Read the model definition and answer for the solid it produces. Units are mm, in the model's axes. Face numbers are marked on the shaded views. A direction names the side the tool comes from. Coordinates: 2 decimals unless noted, no trailing zeros. Write each loop counter-clockwise with the first axis right and the second up, starting at its lowest first coordinate (ties: lowest second). Pieces come first, ordered by that corner, then holes. Notation, with made-up numbers: (43, -6) -> (68, -6) arc R10 ccw to (68, 10) -> close; hole circle Ø6 at (18.5, 40). An arc over 180 degrees is marked (long way). Return JSON: item names as keys, results as strings.
from build123d import *

# Parameters (mm, degrees)
SKETCH1_W           = 58
SKETCH1_H           = 40
BOSS_EXTRUDE1_DEPTH = 22.5
SKETCH2_W           = 8.5
SKETCH2_H           = 17
SKETCH2_R           = 2.15
BOSS_EXTRUDE2_DEPTH = 4.35
FILLET1_R           = 8


with BuildPart() as part:
    # Sketch1 → Boss-Extrude1 (new body)
    with BuildSketch(Plane(origin=(0, 0, 0), x_dir=(1, 0, 0), z_dir=(0, 1, 0))):
        with Locations((29, -20)):
            Rectangle(SKETCH1_W, SKETCH1_H)
    extrude(amount=BOSS_EXTRUDE1_DEPTH)

    # Sketch2 → Boss-Extrude2 (add)
    # profile 1 of 2: a face of its own
    with BuildSketch(Plane(origin=(0, 22.5, 0), x_dir=(1, 0, 0), z_dir=(0, 1, 0))):
        with Locations((62.25, -20)):
            Rectangle(SKETCH2_W, SKETCH2_H)
        with Locations(Location((62.1, -20, 0), (0, 0, 270))):
            Circle(SKETCH2_R, mode=Mode.SUBTRACT)
    # profile 2 of 2: a face of its own
    with BuildSketch(Plane(origin=(0, 22.5, 0), x_dir=(1, 0, 0), z_dir=(0, 1, 0))):
        with Locations((-4.25, -20)):
            Rectangle(SKETCH2_W, SKETCH2_H)
        with Locations(Location((-4.2, -20, 0), (0, 0, 270))):
            Circle(SKETCH2_R, mode=Mode.SUBTRACT)
    extrude(amount=-BOSS_EXTRUDE2_DEPTH)

    # Fillet1
    fillet1_edges = [part.edges().sort_by_distance(p)[0] for p in [
        (66.5, 20.325, 11.5),
        (66.5, 20.325, 28.5),
        (-8.5, 20.325, 28.5),
        (-8.5, 20.325, 11.5),
    ]]
    fillet(fillet1_edges, radius=FILLET1_R)


solid = part.part
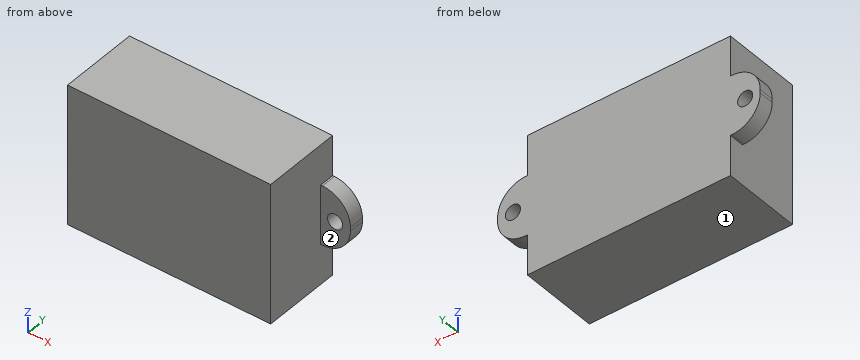
1. The part is cut by section A-A (x = -4.2). Determine the outline of the cut face in (y, z), then the cut area to 3 significant figures.
Taken from the geometry:
{"outline": "(18.15, 12.41) -> (22.5, 12.41) -> (22.5, 17.85) -> (18.15, 17.85) -> close; (18.15, 22.15) -> (22.5, 22.15) -> (22.5, 27.59) -> (18.15, 27.59) -> close", "area": "47.4 mm2"}
2. A tool of negligible diameter and unlimited length cuts with its end or side. For the marked faces 1 and 2, from which of +Z, -Z, +X, -X, +Y, -Y can it reach the whole face along a straight path? Write none if from no direction.
Taken from the geometry:
{"face 1": "-Z, +X, -X, +Y, -Y", "face 2": "+Z, -Z, +X, -Y"}
3. The part is cut by section B-B (z = 13.5). Determine the outline of the cut face in (x, y), then the cut area to 3 significant figures.
Taken from the geometry:
{"outline": "(-5.79, 18.15) -> (0, 18.15) -> (0, 0) -> (58, 0) -> (58, 18.15) -> (63.79, 18.15) -> (63.79, 22.5) -> (-5.79, 22.5) -> close", "area": "1,360 mm2"}
4. The part is cut by section C-C (x = 62.1). Determine the outline of the cut face in (y, z), then the cut area to 3 significant figures.
Taken from the geometry:
{"outline": "(18.15, 12.36) -> (22.5, 12.36) -> (22.5, 17.85) -> (18.15, 17.85) -> close; (18.15, 22.15) -> (22.5, 22.15) -> (22.5, 27.64) -> (18.15, 27.64) -> close", "area": "47.8 mm2"}
5. Consider L1, parallel to X at y = 21.25, z = 20; L2, parallel to X at y = 11.5, z = 2; L3, parallel to Y at x = 61, z = 15.5. Determine where each line is inside the solid, lowest interval first.
Taken from the geometry:
{"L1": "x = -8.5 to -6.35, -2.05 to 59.95, 64.25 to 66.5", "L2": "x = 0 to 58", "L3": "y = 18.15 to 22.5"}
6. Flat-ended cylindrical pins translate along their axes: pin 1 Ø2.5 at (x, z) = (62.1, 20) entering from -Y; pin 2 Ø3 at (y, z) = (6, 15) entering from +X; pin 3 Ø8 at (y, z) = (13.5, 17) entering from -X; pin 4 Ø4.5 at (x, z) = (-4, 17) entering from -Y. Find the tip coordinate at first contact, or state that the pin passes through.
Taken from the geometry:
{"pin 1": "passes through", "pin 2": "stops at x = 58", "pin 3": "stops at x = 0", "pin 4": "stops at y = 18.15"}
7. The part is cut by section D-D (y = 2.25). Determine the outline of the cut face in (x, z), then the cut area to 3 significant figures.
Taken from the geometry:
{"outline": "(0, 0) -> (58, 0) -> (58, 40) -> (0, 40) -> close", "area": "2,320 mm2"}
